Design review of the part shown in the three views and the two pictorial views. Dimensions are in mm from the part's minimum x, y and z. A direction names the side the tool comes from. Give positions to 0.01 mm unless a question says otherwise; leave off trailing zeros. Order: outer loops, then holes, each group sorted by start corner. A loop starts at its lowest first (then second) coordinate and runs counter-clockwise, first axis right, second up. Notation, with made-up numbers: (9.25, 73.5) - (27.25, 73.5) arc R18 cw to (27.25, 101.5) - close; hole circle Ø4 at (6, -18). An arc over 180 degrees is marked (long way). Put each result on its own line as item: value. Start each with the question number.
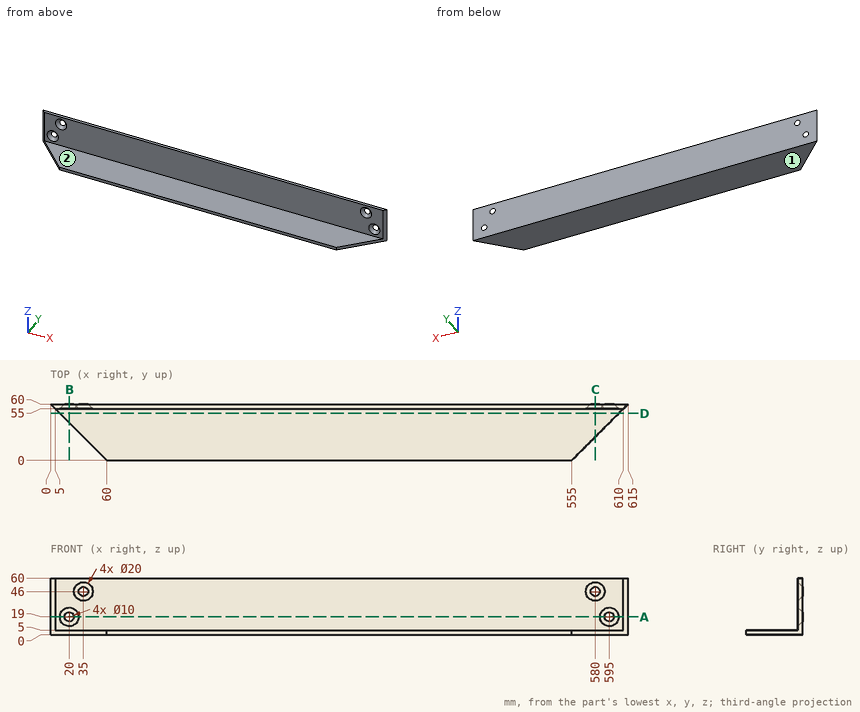
1. Tool access review of the marked faces 1 and 2: name each direction out of +Z, -Z, +X, -X, +Y, -Y from which nothing blocks a thin tool from reaching the whole face with its end or side.
2. Add section D-D, the plane y = 50. Give the boundary of the cut face in (x, z).
3. Clearance check with flat-ended pins moving along their axes: pin 1 (2 mm diameter, centred on x = 153, y = 26.5, fed in from +Z); pin 2 (1.5 mm diameter, centred on x = 205, z = 8.5, fed in from -Y). State where each tip first meets the part, or that it passes through.
4. Add section B-B, the plane x = 20. Give the boundary of the cut face in (y, z), then the cut area to 3 significant figures.
5. Add section A-A, the plane z = 19. Give the boundary of the cut face in (x, y).
6. Add section C-C, the plane x = 580. Give the boundary of the cut face in (y, z), then the cut area to 3 significant figures.
7. Wall thickness on line 1 (Z direction, x = 74.5, y = 54); line 2 (Y direction, x = 416, z = 21); line 3 (X direction, y = 57.5, z = 3): over which ranges is each line inside the solid? List them lowest first. Write a range as from..to.
Found:
1. face 1: -Z, +X, -X, +Y, -Y
1. face 2: +Z, +X, -X, -Y
2. outline: (10, 0) - (605, 0) - (605, 5) - (10, 5) - close
3. pin 1: stops at z = 5
3. pin 2: stops at y = 55
4. outline: (40, 0) - (60, 0) - (60, 14) - (55, 9) - (55, 5) - (40, 5) - close; (55, 29) - (60, 24) - (60, 60) - (55, 60) - close
4. area: 300 mm^2
5. outline: (0, 60) - (5, 55) - (10, 55) - (15, 60) - close; (25, 60) - (30, 55) - (585, 55) - (590, 60) - close; (600, 60) - (605, 55) - (610, 55) - (615, 60) - close
6. outline: (25, 0) - (60, 0) - (60, 41) - (55, 36) - (55, 5) - (25, 5) - close; (55, 56) - (60, 51) - (60, 60) - (55, 60) - close
6. area: 375 mm^2
7. line 1: z = 0..5
7. line 2: y = 55..60
7. line 3: x = 2.5..612.5
